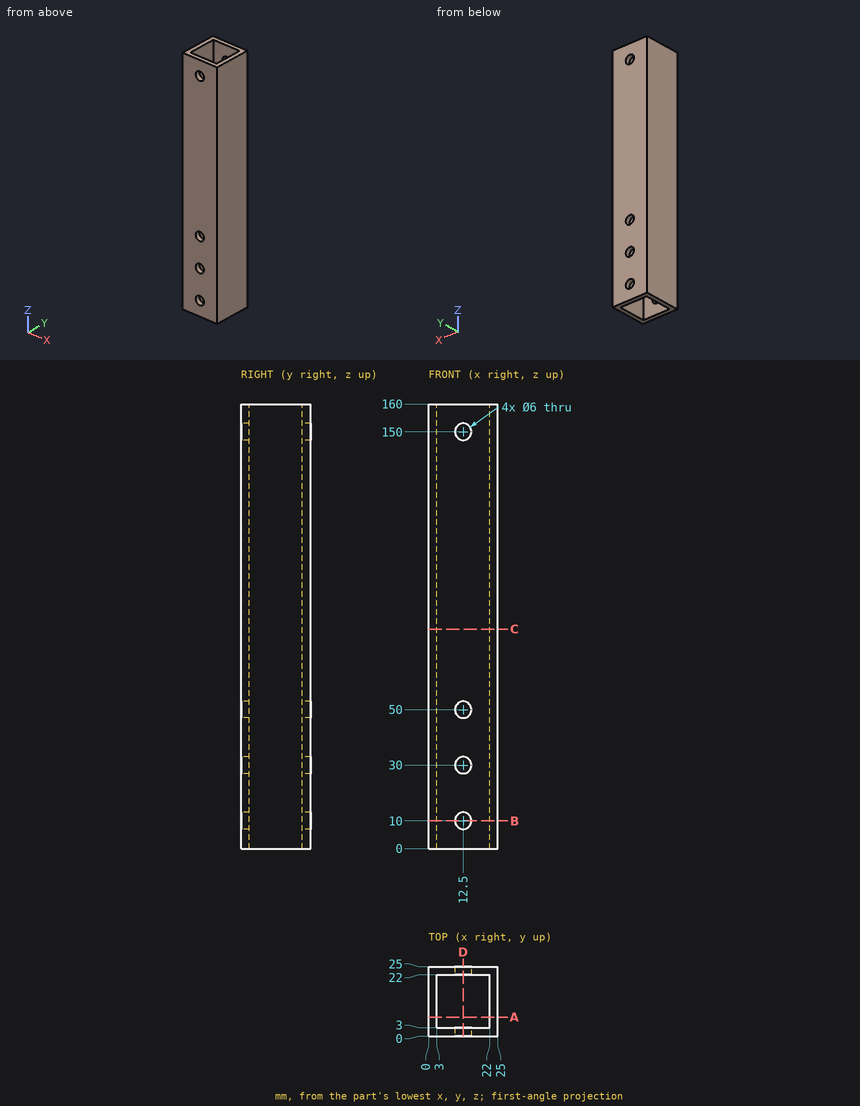
Source: three-view drawing plus pictorial views. Frame: mm from the lowest corner of the part. Give positions to 0.01 mm unless a question says otherwise; leave off trailing zeros. Order: outer loops, then holes, each group sorted by start corner. A loop starts at its lowest first (then second) coordinate and runs counter-clockwise, first axis right, second up. Notation, with made-up numbers: M 80.5,29.5 L 118.5,29.5 A13 cw 118.5,35.5 Z; hole C 8.5,45.5 d3. An arc over 180 degrees is marked long. One line per question, with ' | ' between items. Start each with the question number.
1. Material intervals for probe 1 along Z at (x, y) = (12.5, 24.2); probe 2 along X at (y, z) = (4, 93.5), sorted ascending. Write a range as [from, to].
2. Section query C-C (z = 79). Return the cut outline in (x, y), and give its area (3 significant figures).
3. Section query D-D (x = 12.5). Count the separate pieces of the cut face and the enclosed holes in it, and give its area (3 significant figures).
4. Section query B-B (z = 10). Return the cut outline in (x, y), and give its area (3 significant figures).
5. Section query A-A (y = 6.75). Return the cut outline in (x, z), and give its area (3 significant figures).
Here are the results:
1) probe 1: [0, 7], [13, 27], [33, 47], [53, 147], [153, 160] | probe 2: [0, 3], [22, 25]
2) outline: M 0,0 L 25,0 L 25,25 L 0,25 Z; hole M 3,3 L 22,3 L 22,22 L 3,22 Z | area: 264 mm²
3) separate pieces: 10 | enclosed holes: 0 | area: 816 mm²
4) outline: M 0,0 L 9.5,0 L 9.5,3 L 3,3 L 3,22 L 9.5,22 L 9.5,25 L 0,25 Z; M 15.5,0 L 25,0 L 25,25 L 15.5,25 L 15.5,22 L 22,22 L 22,3 L 15.5,3 Z | area: 228 mm²
5) outline: M 0,0 L 3,0 L 3,160 L 0,160 Z; M 22,0 L 25,0 L 25,160 L 22,160 Z | area: 960 mm²
